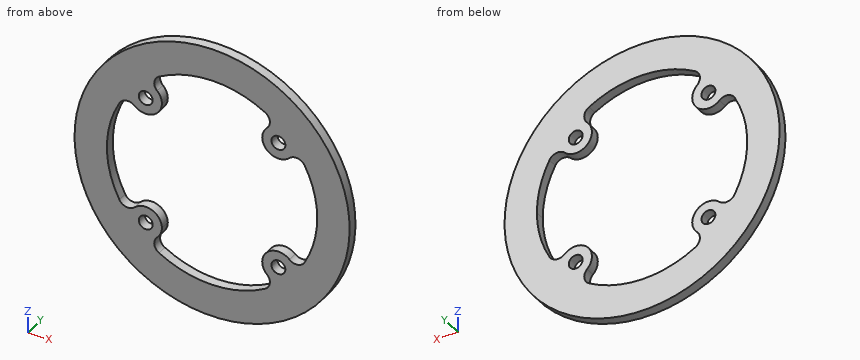
```python
from build123d import *

# Parameters (mm, degrees)
SKETCH_1_R          = 45
SKETCH_1_R_2        = 2
EXTRUDE_1_DEPTH     = 3
CUT_EXTRUDE_1_DEPTH = 64.710281745
FILLET_1_R          = 3
MOVE_FACE_1_BY      = 2.5
MOVE_FACE_2_BY      = 0.15
MOVE_FACE_2_2_BY    = 0.15
MOVE_FACE_2_3_BY    = 0.15
MOVE_FACE_2_4_BY    = 0.15


with BuildPart() as part:
    # ｽｹｯﾁ1 → ﾎﾞｽ - 押し出し1 (new body)
    with BuildSketch(Plane(origin=(0, 0, 0), x_dir=(1, 0, 0), z_dir=(0, 1, 0))):
        with Locations(Location((0, 0, 0), (0, 0, 270))):
            Circle(SKETCH_1_R)
        with Locations(Location((-20.5, -19.798989873, 0), (0, 0, 270))):
            Circle(SKETCH_1_R_2, mode=Mode.SUBTRACT)
        with Locations(Location((20.5, -19.798989873, 0), (0, 0, 90))):
            Circle(SKETCH_1_R_2, mode=Mode.SUBTRACT)
        with Locations(Location((20.5, 19.798989873, 0), (0, 0, 270))):
            Circle(SKETCH_1_R_2, mode=Mode.SUBTRACT)
        with Locations(Location((-20.5, 19.798989873, 0), (0, 0, 90))):
            Circle(SKETCH_1_R_2, mode=Mode.SUBTRACT)
    extrude(amount=EXTRUDE_1_DEPTH)

    # ｽｹｯﾁ2 → ｶｯﾄ - 押し出し1 (cut, through all)
    with BuildSketch(Plane(origin=(0, 3, 0), x_dir=(1, 0, 0), z_dir=(0, 1, 0))):
        with BuildLine():
            ThreePointArc((25.486471606, -20.166550649), (30.696582279, -10.675665619), (32.5, 0))
            ThreePointArc((32.5, 0), (30.696582279, 10.675665619), (25.486471606, 20.166550649))
            ThreePointArc((25.486471606, 20.166550649), (25.496616757, 19.9828947), (25.5, 19.798989873))
            ThreePointArc((25.5, 19.798989873), (16.778183392, 16.460115641), (21.040767545, 24.769660901))
            ThreePointArc((21.040767545, 24.769660901), (0, 32.5), (-21.040767545, 24.769660901))
            ThreePointArc((-21.040767545, 24.769660901), (-17.161125768, 23.520806481), (-15.5, 19.798989873))
            ThreePointArc((-15.5, 19.798989873), (-20.683904827, 14.802373116), (-25.486471606, 20.166550649))
            ThreePointArc((-25.486471606, 20.166550649), (-32.5, 0), (-25.486471606, -20.166550649))
            ThreePointArc((-25.486471606, -20.166550649), (-20.683904827, -14.802373116), (-15.5, -19.798989873))
            ThreePointArc((-15.5, -19.798989873), (-17.161125768, -23.520806481), (-21.040767545, -24.769660901))
            ThreePointArc((-21.040767545, -24.769660901), (0, -32.5), (21.040767545, -24.769660901))
            ThreePointArc((21.040767545, -24.769660901), (16.778183392, -16.460115641), (25.5, -19.798989873))
            ThreePointArc((25.5, -19.798989873), (25.496616757, -19.9828947), (25.486471606, -20.166550649))
        make_face()
    extrude(amount=-CUT_EXTRUDE_1_DEPTH, mode=Mode.SUBTRACT)

    # ﾌｨﾚｯﾄ1
    fillet_1_edges = [part.edges().sort_by_distance(p)[0] for p in [
        (21.040767545, 1.5, -24.769660901),
        (25.486471606, 1.5, -20.166550649),
        (25.486471606, 1.5, 20.166550649),
        (21.040767545, 1.5, 24.769660901),
        (-21.040767545, 1.5, 24.769660901),
        (-25.486471606, 1.5, 20.166550649),
        (-25.486471606, 1.5, -20.166550649),
        (-21.040767545, 1.5, -24.769660901),
    ]]
    fillet(fillet_1_edges, radius=FILLET_1_R)

    # Move Face 1: a curved face moved inward by 2.5
    add(Solid.thicken(part.faces().sort_by_distance((0, 1.5, -45))[0], -MOVE_FACE_1_BY), mode=Mode.SUBTRACT)

    # Move Face 2: a curved face moved inward by 0.15
    add(Solid.thicken(part.faces().sort_by_distance((20.5, 1.5, -21.798989873))[0], -MOVE_FACE_2_BY), mode=Mode.SUBTRACT)

    # Move Face 2 2: a curved face moved inward by 0.15
    add(Solid.thicken(part.faces().sort_by_distance((-20.5, 1.5, -17.798989873))[0], -MOVE_FACE_2_2_BY), mode=Mode.SUBTRACT)

    # Move Face 2 3: a curved face moved inward by 0.15
    add(Solid.thicken(part.faces().sort_by_distance((-20.5, 1.5, 17.798989873))[0], -MOVE_FACE_2_3_BY), mode=Mode.SUBTRACT)

    # Move Face 2 4: a curved face moved inward by 0.15
    add(Solid.thicken(part.faces().sort_by_distance((20.5, 1.5, 21.798989873))[0], -MOVE_FACE_2_4_BY), mode=Mode.SUBTRACT)


solid = part.part
```
CAD build for the part. Positions are in the model's coordinates, mm. Give positions to 0.01 mm unless a question says otherwise; leave off trailing zeros. Write each loop counter-clockwise with the first axis right and the second up, starting at its lowest first coordinate (ties: lowest second). Pieces come first, ordered by that corner, then holes. Notation, with made-up numbers: (-39, 41) -> (-12, 41) arc R23 cw to (-12, 77) -> close; hole circle Ø11 at (-35.75, 65.5). An arc over 180 degrees is marked (long way). Write each question's results on one line, items separated by ' | '.
1. Drop a flat-ended pin along its axis: P1, Ø4, axis at x = 20.5, z = -19.8, coming from the +Y side. Give the stop position or say it passes through.
Geometry check:
P1: through
2. Cut at B-B, the plane z = -11.5. Write the cut outline in (x, y).
Geometry check:
outline: (-40.91, 0) -> (-30.4, 0) -> (-30.4, 3) -> (-40.91, 3) -> close; (30.4, 0) -> (40.91, 0) -> (40.91, 3) -> (30.4, 3) -> close
3. Cut at A-A, the plane x = 0. Write the cut outline in (y, z), then the cut area to 3 significant figures.
Geometry check:
outline: (0, -42.5) -> (3, -42.5) -> (3, -32.5) -> (0, -32.5) -> close; (0, 32.5) -> (3, 32.5) -> (3, 42.5) -> (0, 42.5) -> close | area: 60.0 mm²
4. Cut at C-C, the plane x = -20.5. Write the cut outline in (y, z).
Geometry check:
outline: (0, -37.23) -> (3, -37.23) -> (3, -21.95) -> (0, -21.95) -> close; (0, -17.65) -> (3, -17.65) -> (3, -14.8) -> (0, -14.8) -> close; (0, 14.8) -> (3, 14.8) -> (3, 17.65) -> (0, 17.65) -> close; (0, 21.95) -> (3, 21.95) -> (3, 37.23) -> (0, 37.23) -> close
5. Wall check: probe 1 along X at (y, z) = (0.15, -16); probe 2 along X at (y, z) = (1.8, -18); probe 3 along Z at (x, y) = (-8, 1.05). Give the ranges that are in metal, low to high. Write a range as [from, to].
Geometry check:
probe 1: [-39.37, -28.19], [-23.75, -17.25], [17.25, 23.75], [28.19, 39.37] | probe 2: [-38.5, -21.68], [-19.32, -15.83], [15.83, 19.32], [21.68, 38.5] | probe 3: [-41.74, -31.5], [31.5, 41.74]
6. Cut at D-D, the plane z = -34. Write the cut outline in (x, y).
Geometry check:
outline: (-25.5, 0) -> (25.5, 0) -> (25.5, 3) -> (-25.5, 3) -> close
